Part print with two shaded views. Sizes in mm from the minimum x, y, z corner. A direction names the side the tool comes from. Give positions to 0.01 mm unless a question says otherwise; leave off trailing zeros. Write each loop counter-clockwise with the first axis right and the second up, starting at its lowest first coordinate (ties: lowest second). Pieces come first, ordered by that corner, then holes.
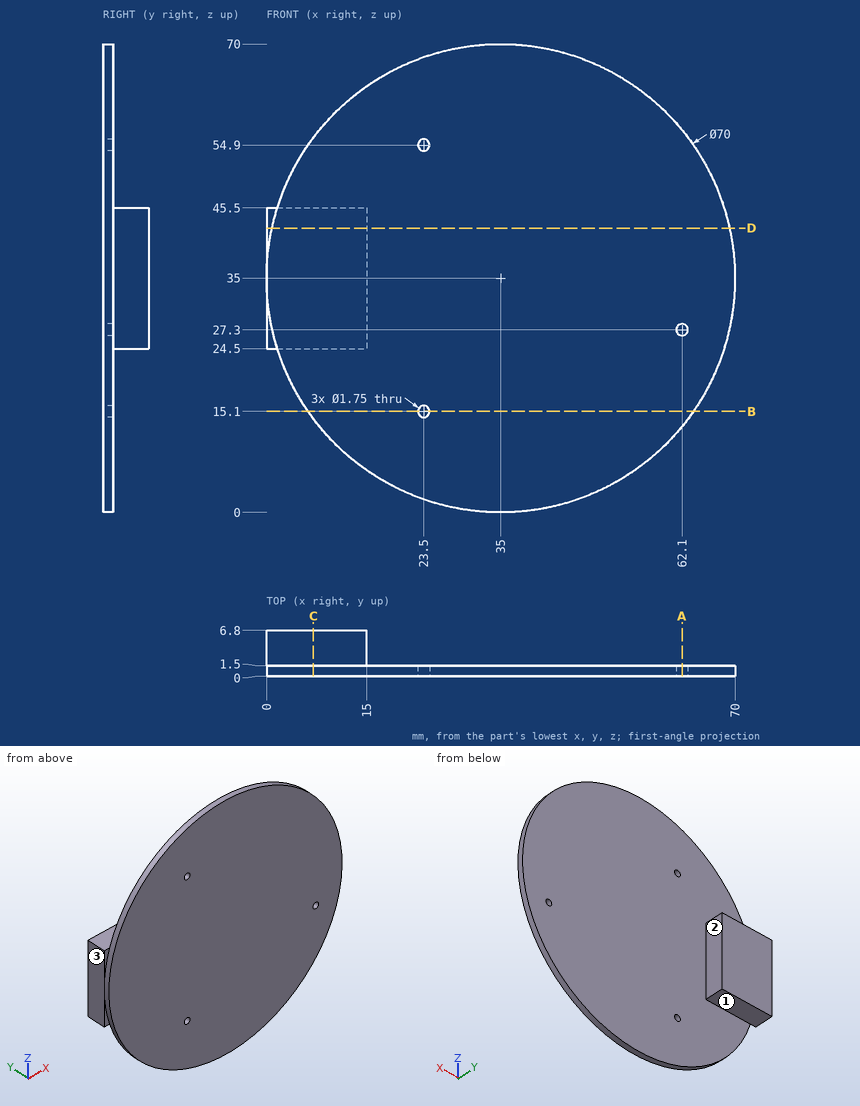
1) Flat gauge pins, fed straight in: P1, Ø2.5, axis at x = 62.1, z = 27.3, coming from the +Y side; P2, Ø2.5, axis at x = 6.5, y = 3.5, coming from the -Z side; P3, Ø2.5, axis at y = 3, z = 31.5, coming from the +X side. Where does each tip first touch, or does it go through?
Check result:
P1: stops at y = 1.5
P2: stops at z = 24.5
P3: stops at x = 15
2) Saw through at A-A (x = 62.1). Write the cut outline in (y, z) (3 decimals), and give its area (3 significant figures).
Check result:
outline: (0, 12.851) - (1.5, 12.851) - (1.5, 26.425) - (0, 26.425) - close; (0, 28.175) - (1.5, 28.175) - (1.5, 57.149) - (0, 57.149) - close
area: 63.8 mm2
3) Drill centre lines: L1, parallel to Y at x = 60, z = 53; L2, parallel to X at y = 0.45, z = 27.3 (1 decimal); L3, parallel to Z at x = 8, y = 2.75. Where is each one in solid material? Low to high.
Check result:
L1: y = 0 to 1.5
L2: x = 0.9 to 61.2, 63 to 69.1
L3: z = 24.5 to 45.5
4) Saw through at B-B (z = 15.1). Write the cut outline in (x, y) (3 decimals), and give its area (3 significant figures).
Check result:
outline: (6.208, 0) - (22.625, 0) - (22.625, 1.5) - (6.208, 1.5) - close; (24.375, 0) - (63.792, 0) - (63.792, 1.5) - (24.375, 1.5) - close
area: 83.8 mm2
5) Saw through at C-C (x = 7). Write the cut outline in (y, z).
Check result:
outline: (0, 14) - (1.5, 14) - (1.5, 24.5) - (6.8, 24.5) - (6.8, 45.5) - (1.5, 45.5) - (1.5, 56) - (0, 56) - close
6) Saw through at D-D (z = 42.5). Write the cut outline in (x, y).
Check result:
outline: (0, 1.5) - (0.81, 1.5) - (0.81, 0) - (69.19, 0) - (69.19, 1.5) - (15, 1.5) - (15, 6.8) - (0, 6.8) - close
7) 3-axis set-ups, long thin cutter, end or side, ignore diameter. For the marked faces 1, 2 and 3: which of +Z, -Z, +X, -X, +Y, -Y reach the whole face in a straight line?
Check result:
face 1: -Z, +X, -X, +Y
face 2: +Z, -Z, +X, +Y
face 3: +Z, -Z, -X, +Y, -Y
